Source: CAD feature listing. Evaluate the final solid. Frame: model axes, mm. Give positions to 0.01 mm unless a question says otherwise; leave off trailing zeros. Loops run counter-clockwise (first coordinate to the right, second up) from the corner with the lowest first, then second, coordinate; pieces in that order, holes last. Notation, with made-up numbers: M 3.5,77 L 37.5,77 A23 cw 37.5,116 Z; hole C 46,3.5 d2. An arc over 180 degrees is marked long. Answer in a Markdown table with one row per item.
```python
from build123d import *

# Parameters (mm, degrees)
EXTRUDE_1_DEPTH = 6


with BuildPart() as part:
    # 草图1 → 凸台-拉伸1 (new body)
    with BuildSketch(Plane.XY):
        with BuildLine():
            Line((-5.38, 7.694214332), (-5.38, -120.055785668))
            ThreePointArc((-5.38, -120.055785668), (-6.771242789, -123.414542878), (-10.13, -124.805785668))
            Line((-10.13, -124.805785668), (-137.202114628, -124.805785668))
            ThreePointArc((-137.202114628, -124.805785668), (-141.48, -130.152309812), (-137.202114628, -135.498833956))
            Line((-137.202114628, -135.498833956), (-10.13, -135.498833956))
            ThreePointArc((-10.13, -135.498833956), (-6.771242789, -136.890076745), (-5.38, -140.248833956))
            Line((-5.38, -140.248833956), (-5.38, -267.998833956))
            ThreePointArc((-5.38, -267.998833956), (0, -273.378833956), (5.38, -267.998833956))
            Line((5.38, -267.998833956), (5.38, -140.248833956))
            ThreePointArc((5.38, -140.248833956), (6.771242789, -136.890076745), (10.13, -135.498833956))
            Line((10.13, -135.498833956), (137.202114628, -135.498833956))
            ThreePointArc((137.202114628, -135.498833956), (141.48, -130.152309812), (137.202114628, -124.805785668))
            Line((137.202114628, -124.805785668), (10.13, -124.805785668))
            ThreePointArc((10.13, -124.805785668), (6.771242789, -123.414542878), (5.38, -120.055785668))
            Line((5.38, -120.055785668), (5.38, 7.694214332))
            ThreePointArc((5.38, 7.694214332), (0, 13.074214332), (-5.38, 7.694214332))
        make_face()
        with BuildLine():
            Line((-4.75, 7.694214332), (-4.75, -120.055785668))
            ThreePointArc((-4.75, -120.055785668), (-6.325765517, -123.860020151), (-10.13, -125.435785668))
            Line((-10.13, -125.435785668), (-137.13, -125.435785668))
            ThreePointArc((-137.13, -125.435785668), (-140.85, -130.152309812), (-137.13, -134.868833956))
            Line((-137.13, -134.868833956), (-10.13, -134.868833956))
            ThreePointArc((-10.13, -134.868833956), (-6.325765517, -136.444599473), (-4.75, -140.248833956))
            Line((-4.75, -140.248833956), (-4.75, -267.998833956))
            ThreePointArc((-4.75, -267.998833956), (0, -272.748833956), (4.75, -267.998833956))
            Line((4.75, -267.998833956), (4.75, -140.248833956))
            ThreePointArc((4.75, -140.248833956), (6.325765517, -136.444599473), (10.13, -134.868833956))
            Line((10.13, -134.868833956), (137.13, -134.868833956))
            ThreePointArc((137.13, -134.868833956), (140.85, -130.152309812), (137.13, -125.435785668))
            Line((137.13, -125.435785668), (10.13, -125.435785668))
            ThreePointArc((10.13, -125.435785668), (6.325765517, -123.860020151), (4.75, -120.055785668))
            Line((4.75, -120.055785668), (4.75, 7.694214332))
            ThreePointArc((4.75, 7.694214332), (0, 12.444214332), (-4.75, 7.694214332))
        make_face(mode=Mode.SUBTRACT)
    extrude(amount=EXTRUDE_1_DEPTH)


solid = part.part
```
1) Pin query (flat end, axial travel): pin 1 Ø1.8 at (x, z) = (-98, 3) entering from +Y; pin 2 Ø3 at (y, z) = (-234.5, 3) entering from +X; pin 3 Ø1.8 at (y, z) = (-225.5, 2.5) entering from -X. Return the tip coordinate at first contact, or that it passes through.
Reply:
| item | result |
|---|---|
| pin 1 | stops at y = -124.81 |
| pin 2 | stops at x = 5.38 |
| pin 3 | stops at x = -5.38 |
2) Material intervals for L1, parallel to X at y = -25.5, z = 2.55; L2, parallel to Y at x = -52, z = 5.75, sorted ascending.
Reply:
| item | result |
|---|---|
| L1 | x = -5.38 to -4.75, 4.75 to 5.38 |
| L2 | y = -135.5 to -134.87, -125.44 to -124.81 |
3) Section A-A, the plane y = -249. Return loops of the section in (x, z), then the cut area to 3 significant figures.
Reply:
| item | result |
|---|---|
| outline | M -5.38,0 L -4.75,0 L -4.75,6 L -5.38,6 Z; M 4.75,0 L 5.38,0 L 5.38,6 L 4.75,6 Z |
| area | 7.56 mm² |
4) Section C-C, the plane x = 0. Return loops of the section in (y, z).
Reply:
| item | result |
|---|---|
| outline | M -273.38,0 L -272.75,0 L -272.75,6 L -273.38,6 Z; M 12.44,0 L 13.07,0 L 13.07,6 L 12.44,6 Z |
